Autodesk Inventor part; units mm, degrees
ref_plane "Work Plane2" through (-16.1743, -15.6151, -101.1913) normal (0, 0, -1) x (0, 1, 0)
ref_plane "YZ Plane" through (0, 0, 0) normal (1, 0, 0) x (0, 1, 0)
ref_plane "XZ Plane" through (0, 0, 0) normal (0, 1, 0) x (-1, 0, 0)
ref_plane "Work Plane1" through (-17.3808, -12.8161, -79.6267) normal (0, 0, 1) x (1, 0, 0)
sketch "Sketch2" plane through (-17.3808, -12.8161, -79.6267) normal (0, 0, 1) x (1, 0, 0)
  circle A0 centre (0, 0) radius 3.175
  line L0 (2.7795, -1.5347) -> (0.0606, -3.1744)
  line L1 (0.0606, -3.1744) -> (-2.7188, -1.6397)
  line L2 (-2.7188, -1.6397) -> (-2.7795, 1.5347)
  line L3 (-2.7795, 1.5347) -> (-0.0606, 3.1744)
  line L4 (-0.0606, 3.1744) -> (2.7188, 1.6397)
  line L5 (2.7188, 1.6397) -> (2.7795, -1.5347)
  point P0 (17.3808, 12.8161)
ref_plane "Work Plane2" through (-16.1743, -15.6151, -101.1913) normal (0, 0, -1) x (0, 1, 0)
extrude "Extrusion1" add sketch "Sketch2" against normal up to surface (21.5646 mm away) contours L5 L0 L1 L2 L3 L4
properties part number "ArmSolenoidShaftBoundingBox"
Model file for the job. Use its own axes, mm. Coordinates: 2 decimals unless noted, no trailing zeros. Loops run counter-clockwise (first coordinate to the right, second up) from the corner with the lowest first, then second, coordinate; pieces in that order, holes last. Notation, with made-up numbers: M 56,-12 L 77,-12 A17 ccw 77,9 Z; hole C -29,-8.75 d7. An arc over 180 degrees is marked long. Use CSV: the item, a comma, the result in double quotes. Start each with the question number.
1. Probe probe 1 along X at (y, z) = (-14.25, -97); probe 2 along Y at (x, z) = (-17.3, -90.75); probe 3 along Y at (x, z) = (-15.7, -99.75). List the from-to ranges inside material, lowest first. Write a range as [from, to].
2. Flat gauge pin, fed straight in: pin 1 (1 mm diameter, centred on y = -13, z = -97, fed in from -X). Where does the tip first touch, or does it go through?
3. Band-saw the part on B-B, the plane y = -10. List the corners of the cut face in (x, z).
4. Band-saw the part on C-C, the plane x = -17.95. List the corners of the cut face in (y, z).
5. Band-saw the part on A-A, the plane z = -96.25. List the corners of the cut face in (x, y), then the cut area to 3 significant figures.
Entries:
1,probe 1,"x = [-20.1, -14.6]"
1,probe 2,"y = [-15.98, -9.72]"
1,probe 3,"y = [-15.01, -10.6]"
2,pin 1,"stops at x = -20.14"
3,outline,"M -18.04,-101.19 L -16.79,-101.19 L -16.79,-79.63 L -18.04,-79.63 Z"
4,outline,"M -15.64,-101.19 L -9.95,-101.19 L -9.95,-79.63 L -15.64,-79.63 Z"
5,outline,"M -20.16,-11.28 L -20.1,-14.46 L -17.32,-15.99 L -14.6,-14.35 L -14.66,-11.18 L -17.44,-9.64 Z"
5,area,"26.2 mm2"
